Autodesk Inventor part; units mm, degrees
ref_plane "YZ Plane" through (0, 0, 0) normal (1, 0, 0) x (0, 1, 0)
ref_plane "XZ Plane" through (0, 0, 0) normal (0, 1, 0) x (-1, 0, 0)
ref_plane "XY Plane" through (0, 0, 0) normal (0, 0, 1) x (1, 0, 0)
sketch "Эскиз1" plane through (0, 0, 0) normal (1, 0, 0) x (0, 1, 0)
  circle A0 centre (35.2311, -22.6062) radius 9.3
  circle A1 centre (0, -38.8201) radius 6.1 construction
  circle A2 centre (0, 0) radius 4.85 construction
  circle A3 centre (35.8147, -49.5529) radius 3.55
  line L0 (6.0968, -38.6237) -> (4.8475, 0.1562) construction
  line L1 (-4.8475, 0.1562) -> (-6.0968, -38.6237) construction
  line L2 (0, 0) -> (0, -38.8201) construction
  circle A4 centre (0, -38.8201) radius 4.1
  circle A5 centre (0, 0) radius 2.25
  circle A6 centre (0, -38.8201) radius 15 construction
  circle A7 centre (0, 0) radius 14 construction
  circle A8 centre (0, -38.8201) radius 7.6
  circle A9 centre (0, 0) radius 7 construction
  line L3 (7.5465, -39.7207) -> (12.114, -1.4456)
  line L4 (-7.5465, -39.7207) -> (-12.114, -1.4456)
  circle A10 centre (0, 0) radius 8.8 construction
  circle A11 centre (0, 0) radius 12.2
  circle A12 centre (6.8983, -19.8347) radius 1.6
  circle A13 centre (-7.3019, -16.4524) radius 1.6
  point P0 (-7, 0)
  point P1 (-7.5465, -39.7207)
  point P2 (-12.114, -1.4456)
  dimension "d0" = 18.6
  dimension "d1" = 12.2
  dimension "d2" = 9.7
  dimension "d3" = 7.1
  dimension "d8" = 38.8201
  dimension "d13" = 38.8
  dimension "d14" = 38.8
  dimension "d23" = 8.2
  dimension "d24" = 4.5
  dimension "d25" = 30
  dimension "d26" = 28
  dimension "d28" = 14
  dimension "d31" = 17.6
  dimension "d32" = 3.4
  dimension "d56" = 3.5
  dimension "d58" = 3.2
  dimension "d59" = 3
  dimension "d60" = 21
  dimension "d61" = 3.2
  dimension "d62" = 3
  dimension "d63" = 18
extrude "Выдавливание4" add sketch "Эскиз1" along normal blind 3 contours A5 | A8 | A8 L4 A11 L3 | A11
sketch "Эскиз4" plane through (0, 0, 0) normal (-1, 0, 0) x (0, 0, 1)
  circle A0 centre (-6.2, 6.2) radius 1.4
  circle A1 centre (-38.8201, 0) radius 4.1 construction
  arc A2 (-1.4456, -12.114) -> (-1.4456, 12.114) centre (0, 0) ccw construction
  line L0 (-39.7207, 7.5465) -> (-1.4456, 12.114) construction
  arc A3 (-39.7207, 7.5465) -> (-39.7207, -7.5465) centre (-38.8201, 0) ccw construction
  line L1 (-1.4456, -12.114) -> (-39.7207, -7.5465) construction
  line L2 (0, 0) -> (0, 12.2) construction
  arc A4 (-1.4456, -12.114) -> (-1.4456, 12.114) centre (0, 0) ccw construction
  line L3 (0, 0) -> (12.2, 0) construction
  circle A5 centre (6.2, 6.2) radius 1.4
  circle A6 centre (-6.2, -6.2) radius 1.4
  circle A7 centre (6.2, -6.2) radius 1.4
  dimension "d33" = 2.8
  dimension "d34" = 12.4
  dimension "d35" = 12.4
extrude "Выдавливание5" [suppressed]
sketch "Эскиз5" plane through (3, 0, 0) normal (1, 0, 0) x (0, 0, -1)
  circle A0 centre (0, 0) radius 3.75
  dimension "d38" = 7.5
extrude "Выдавливание6" [suppressed]
sketch "Эскиз6" plane through (3, 0, 0) normal (1, 0, 0) x (0, 0, -1)
  circle A0 centre (0, -18) radius 2
  circle A1 centre (38.8201, 0) radius 4.1 construction
  line L0 (39.7207, 7.5465) -> (1.4456, 12.114) construction
  arc A2 (1.4456, 12.114) -> (1.4456, -12.114) centre (0, 0) ccw construction
  line L1 (1.4456, -12.114) -> (39.7207, -7.5465) construction
  arc A3 (39.7207, -7.5465) -> (39.7207, 7.5465) centre (38.8201, 0) ccw construction
  line L2 (0, 0) -> (0, -26.6004) construction
  circle A4 centre (0, 0) radius 14 construction
  line L3 (-10.8605, -5.5578) -> (-3.5608, -19.8222)
  arc A5 (0, -14) -> (-3.5608, -19.8222) centre (0, -18) ccw construction
  line L4 (2.8284, -20.8284) -> (12.911, -10.7458)
  line L5 (1.4456, -12.114) -> (39.7207, -7.5465) construction
  arc A6 (2.8284, -20.8284) -> (0, -14) centre (0, -18) ccw construction
  arc A7 (-3.5608, -19.8222) -> (2.8284, -20.8284) centre (0, -18) ccw
  line L6 (-10.8605, -5.5578) -> (-10.1465, -5.5578)
  line L7 (-10.1465, -5.5578) -> (-6.8136, -9.4237)
  line L8 (-6.8136, -9.4237) -> (5.1237, -10.512)
  line L9 (5.1237, -10.512) -> (12.911, -10.7458)
  dimension "d42" = 28
  dimension "d41" = 4
  dimension "d43" = 18
  dimension "d44" = 8
  dimension "d45" = 45
extrude "Выдавливание7" [suppressed]
sketch "Эскиз7" plane through (3, 0, 0) normal (1, 0, 0) x (0, 0, -1)
  line L0 (0, 0) -> (0, -29.4139) construction
  circle A0 centre (-9, -15.5885) radius 4.15
  line L1 (-9, -15.5885) -> (0, 0) construction
  circle A1 centre (0, 0) radius 14 construction
  circle A2 centre (0, 0) radius 18 construction
  arc A3 (-5.675, -21.3475) -> (-15.5037, -14.2012) centre (-9, -15.5885) ccw construction
  circle A4 centre (38.8201, 0) radius 4.1 construction
  line L2 (39.7207, 7.5465) -> (1.4456, 12.114) construction
  arc A5 (1.4456, 12.114) -> (1.4456, -12.114) centre (0, 0) ccw
  line L3 (1.4456, -12.114) -> (39.7207, -7.5465)
  arc A6 (39.7207, -7.5465) -> (39.7207, 7.5465) centre (38.8201, 0) ccw construction
  line L4 (-11.9316, 2.5451) -> (-15.5037, -14.2012)
  line L5 (-5.675, -21.3475) -> (12.6295, -10.7794)
  line L6 (1.4456, -12.114) -> (39.7207, -7.5465) construction
  arc A7 (-15.5037, -14.2012) -> (-5.675, -21.3475) centre (-9, -15.5885) ccw
  circle A8 centre (-9, -15.5885) radius 2.75
  dimension "d48" = 8.3
  dimension "d49" = 330
  dimension "d50" = 28
  dimension "d51" = 4
  dimension "d53" = 30
  dimension "d57" = 2.5
  dimension "d64" = 5.5
extrude "Выдавливание8" add sketch "Эскиз7" against normal up to surface (3 mm away) contours A5 L3 L5 A7 L4
extrude "Выдавливание9" add sketch "Эскиз7" against normal up to surface (3 mm away) contours A0
extrude "Выдавливание10" cut sketch "Эскиз7" against normal blind 2.3 contours A0
properties part number "_3DПЕЧАТЬ"
Source: CAD feature listing. Evaluate the final solid. Frame: model axes, mm. A direction names the side the tool comes from. Coordinates: 2 decimals unless noted, no trailing zeros. Loops run counter-clockwise (first coordinate to the right, second up) from the corner with the lowest first, then second, coordinate; pieces in that order, holes last. Notation, with made-up numbers: M 19,-34.5 L 43,-34.5 A8 cw 43,-19.5 Z; hole C -36.75,87 d5. An arc over 180 degrees is marked long. Answer in a Markdown table with one row per item.
Q1. Section A-A on z = 10.5. Return the cut outline in (x, y), plus the area to 3 significant figures.
Answers below:
| item | result |
|---|---|
| outline | M 0,-22.07 L 3,-22.07 L 3,-19.46 L 0.7,-19.46 L 0.7,-17.89 L 0,-17.89 Z; M 0,-13.28 L 0.7,-13.28 L 0.7,-11.72 L 3,-11.72 L 3,6.21 L 0,6.21 Z |
| area | 63.8 mm^2 |
Q2. Draft query along Z for faces 1 (the flat face through (0.7, -16, 6)), 2 (the cylindrical face through (1.5, -20.9, 13)), 3 (the flat face through (1.48, -9.14, -26.36)). Return one class per face: pulls with the +Z half, pulls with the -Z half, needs draft (parallel to the pull), parting line crosses it, or undercut.
Answers below:
| item | result |
|---|---|
| face 1 | undercut |
| face 2 | parting line crosses it |
| face 3 | pulls with the -Z half |
Q3. Set-up query: faces 4 (the cylindrical face through (0.355, -18.028, 7.731)), 5 (the cylindrical face through (1.866, -12.784, 12.059)). Return all of +Z, -Z, +X, -X, +Y, -Y with unobstructed straight access to the full face (end or side cutting, diameter ignored); none if empty.
Answers below:
| item | result |
|---|---|
| face 4 | +X, -X |
| face 5 | +X |
Q4. First-contact query: pin 1 (1 mm diameter, centred on x = 1.5, z = -33.5, fed in from +Y); pin 2 (1.5 mm diameter, centred on x = 2.5, z = -24, fed in from -Y). Flat tips, straight axial feed; report the tip coordinate or a pass-through.
Answers below:
| item | result |
|---|---|
| pin 1 | stops at y = 8.35 |
| pin 2 | stops at y = -9.51 |
Q5. Ray query, probe 1 along Z at (x, y) = (2.85, 2.5); probe 2 along Z at (x, y) = (1.6, 0); probe 3 along Y at (x, z) = (1.65, 10). Return the intervals inside material, ascending. Write a range as from..to.
Answers below:
| item | result |
|---|---|
| probe 1 | z = -46..-42.07, -35.57..11.94 |
| probe 2 | z = -46.42..-42.92, -34.72..12.47 |
| probe 3 | y = -22.16..-19.62, -11.56..6.99 |
Q6. Section D-D on z = -25. Return the cut outline in (x, y), plus the area to 3 significant figures.
Answers below:
| item | result |
|---|---|
| outline | M 0,-9.3 L 3,-9.3 L 3,9.3 L 0,9.3 Z |
| area | 55.8 mm^2 |
Q7. Section C-C on y = 6. Return the cut outline in (x, z).
Answers below:
| item | result |
|---|---|
| outline | M 0,-43.48 L 3,-43.48 L 3,-21.16 L 0,-21.16 Z; M 0,-18.51 L 3,-18.51 L 3,10.62 L 0,10.62 Z |
Q8. Section B-B on y = -0.5. Return the cut outline in (x, z), plus the area to 3 significant figures.
Answers below:
| item | result |
|---|---|
| outline | M 0,-46.4 L 3,-46.4 L 3,-42.89 L 0,-42.89 Z; M 0,-34.75 L 3,-34.75 L 3,12.58 L 0,12.58 Z |
| area | 153 mm^2 |
